```python
from build123d import *

# Parameters (mm, degrees)
SZKIC2_W                         = 60
SZKIC2_H                         = 51.228721397
DODANIE_WYCI_GNI_CIE1_DEPTH      = 40
DODANIE_WYCI_GNI_CIE1_DEPTH_BACK = 30
SZKIC3_R                         = 8.4
WYTNIJ_WYCI_GNI_CIE1_DEPTH       = 52.228721397
SZKIC5_R                         = 17.5
WYTNIJ_WYCI_GNI_CIE2_DEPTH       = 10
SZKIC6_W                         = 5
SZKIC6_H                         = 53
WYTNIJ_WYCI_GNI_CIE3_DEPTH       = 55
SZKIC8_R                         = 22.5
SZKIC8_R_2                       = 17.5
DODANIE_WYCI_GNI_CIE3_DEPTH      = 25


with BuildPart() as part:
    # Szkic2 → Dodanie-wyciągnięcie1 (new body, two sides)
    with BuildSketch(Plane(origin=(0, 0, 0), x_dir=(1, 0, 0), z_dir=(0, 1, 0))) as dodanie_wyci_gni_cie1_sk:
        with Locations((0, 39.614360699)):
            Rectangle(SZKIC2_W, SZKIC2_H)
    extrude(amount=DODANIE_WYCI_GNI_CIE1_DEPTH)
    extrude(dodanie_wyci_gni_cie1_sk.sketch, amount=-DODANIE_WYCI_GNI_CIE1_DEPTH_BACK)

    # Szkic3 → Wytnij-wyciągnięcie1 (cut, through all)
    with BuildSketch(Plane.XY.offset(-14)):
        Circle(SZKIC3_R)
    extrude(amount=-WYTNIJ_WYCI_GNI_CIE1_DEPTH, mode=Mode.SUBTRACT)

    # Szkic5 → Wytnij-wyciągnięcie2 (cut)
    with BuildSketch(Plane(origin=(0, 0, -65.228721397), x_dir=(-1, 0, 0), z_dir=(0, 0, -1))):
        Circle(SZKIC5_R)
    wytnij_wyci_gni_cie2 = extrude(amount=-WYTNIJ_WYCI_GNI_CIE2_DEPTH, mode=Mode.SUBTRACT)

    # Szkic6 → Wytnij-wyciągnięcie3 (cut)
    with BuildSketch(Plane.ZY.offset(30)):
        with Locations((-57.728721397, 0)):
            Rectangle(SZKIC6_W, SZKIC6_H)
    wytnij_wyci_gni_cie3 = extrude(amount=-WYTNIJ_WYCI_GNI_CIE3_DEPTH, mode=Mode.SUBTRACT)

    # Lustro1: Wytnij-wyciągnięcie2, Wytnij-wyciągnięcie3 across plane
    add(wytnij_wyci_gni_cie2.mirror(Plane(origin=(0, 0, -39.614360698), x_dir=(1, 0, 0), z_dir=(0, 0, -1))), mode=Mode.SUBTRACT)
    add(wytnij_wyci_gni_cie3.mirror(Plane(origin=(0, 0, -39.614360698), x_dir=(1, 0, 0), z_dir=(0, 0, -1))), mode=Mode.SUBTRACT)

    # Szkic8 → Dodanie-wyciągnięcie3 (add)
    with BuildSketch(Plane(origin=(0, 0, -65.228721397), x_dir=(-1, 0, 0), z_dir=(0, 0, -1))):
        Circle(SZKIC8_R)
        Circle(SZKIC8_R_2, mode=Mode.SUBTRACT)
    extrude(amount=DODANIE_WYCI_GNI_CIE3_DEPTH)


solid = part.part
```
Design review of the part built by this model. Coordinates are the model's own, in mm. A direction names the side the tool comes from. Give positions to 0.01 mm unless a question says otherwise; leave off trailing zeros. Write each loop counter-clockwise with the first axis right and the second up, starting at its lowest first coordinate (ties: lowest second). Pieces come first, ordered by that corner, then holes.
(1) Tool access review of faces 1 (the face through (-10.382, -19.961, -77.554)), 2 (the face through (-3, 26.5, -21)), 3 (the face through (30, 5, -39)), 4 (the face through (0, -30, -40)), 5 (the face through (13.887, -10.648, -16.465)): name each direction out of +Z, -Z, +X, -X, +Y, -Y from which nothing blocks a thin tool from reaching the whole face with its end or side.
Checked values:
face 1: -Z
face 2: -X
face 3: +Z, -Z, +X, +Y, -Y
face 4: +Z, -Z, +X, -X, -Y
face 5: +Z
(2) Add section A-A (x = 0). Give the boundary of the cut face in (y, z), and give its area (3 significant figures).
Checked values:
outline: (-30, -65.23) - (-22.5, -65.23) - (-22.5, -90.23) - (-17.5, -90.23) - (-17.5, -60.23) - (-26.5, -60.23) - (-26.5, -55.23) - (-8.4, -55.23) - (-8.4, -24) - (-26.5, -24) - (-26.5, -19) - (-17.5, -19) - (-17.5, -14) - (-30, -14) - close; (8.4, -55.23) - (26.5, -55.23) - (26.5, -60.23) - (17.5, -60.23) - (17.5, -90.23) - (22.5, -90.23) - (22.5, -65.23) - (40, -65.23) - (40, -14) - (17.5, -14) - (17.5, -19) - (26.5, -19) - (26.5, -24) - (8.4, -24) - close
area: 2,430 mm2
(3) Mouldability with a two-part tool opening along X and no side actions: class faces 6 (the face through (8.012, 2.523, -39.396)), 7 (the face through (25, 0, -58)), 8 (the face through (-14, 21, -65.229)) as +X half, -X half, draft (parallel to the pull), parting line (faces both ways), or undercut.
Checked values:
face 6: undercut
face 7: -X half
face 8: draft
(4) Clearance check with flat-ended pins moving along their axes: pin 1 Ø2 at (x, y) = (15.5, 0) entering from -Z; pin 2 Ø2.5 at (y, z) = (9.5, -22.5) entering from -X; pin 3 Ø4 at (x, y) = (4, -3.5) entering from -Z; pin 4 Ø8 at (y, z) = (8.5, -72.5) entering from +X. State where each tip first meets the part, or that it passes through.
Checked values:
pin 1: stops at z = -55.23
pin 2: stops at x = 25
pin 3: passes through
pin 4: stops at x = 22.05
(5) Add section C-C (z = -22). Give the boundary of the cut face in (x, y), and give its area (4 significant figures).
Checked values:
outline: (-30, -30) - (30, -30) - (30, 40) - (-30, 40) - (-30, 26.5) - (25, 26.5) - (25, -26.5) - (-30, -26.5) - close
area: 1,285 mm2
(6) Add section B-B (y = -24.5). Give the boundary of the cut face in (x, z).
Checked values:
outline: (-30, -65.23) - (30, -65.23) - (30, -14) - (-30, -14) - (-30, -19) - (25, -19) - (25, -24) - (-30, -24) - (-30, -55.23) - (25, -55.23) - (25, -60.23) - (-30, -60.23) - close
(7) Wall thickness on line 1 along Z through (x, y) = (6.5, -21.5); line 2 along Z through (x, y) = (23, -12); line 3 along Y through (x, z) = (0, -16.2): over which ranges is each line inside the solid? List them lowest first.
Checked values:
line 1: z = -90.23 to -60.23, -55.23 to -24, -19 to -14
line 2: z = -65.23 to -60.23, -55.23 to -24, -19 to -14
line 3: y = -30 to -17.5, 17.5 to 40
(8) Add section D-D (y = 0). Give the boundary of the cut face in (x, z).
Checked values:
outline: (-30, -65.23) - (-22.5, -65.23) - (-22.5, -90.23) - (-17.5, -90.23) - (-17.5, -60.23) - (-30, -60.23) - close; (-30, -55.23) - (-8.4, -55.23) - (-8.4, -24) - (-30, -24) - close; (-30, -19) - (-17.5, -19) - (-17.5, -14) - (-30, -14) - close; (8.4, -55.23) - (25, -55.23) - (25, -60.23) - (17.5, -60.23) - (17.5, -90.23) - (22.5, -90.23) - (22.5, -65.23) - (30, -65.23) - (30, -14) - (17.5, -14) - (17.5, -19) - (25, -19) - (25, -24) - (8.4, -24) - close
